Geometry: final body of the model. Coordinates: model frame, mm. Face numbers are marked on the shaded views. A direction names the side the tool comes from. Give positions to 0.01 mm unless a question says otherwise; leave off trailing zeros. Order: outer loops, then holes, each group sorted by start corner. A loop starts at its lowest first (then second) coordinate and runs counter-clockwise, first axis right, second up. Notation, with made-up numbers: (71, -13) - (83, -13) arc R7 ccw to (83, 0) - close; hole circle Ø7 at (27, 60). An arc over 180 degrees is marked (long way). Put each result on its own line as item: value. Start each with the question number.
1. Section B-B on z = 6. Return the cut outline in (x, y).
2. Section C-C on x = -807.5. Return the cut outline in (y, z).
3. Section A-A on y = -61. Return the cut outline in (x, z).
4. Ray query, line 1 along X through (y, z) = (-70.5, -0.5); line 2 along Y through (x, z) = (-773, -41); line 3 along Y through (x, z) = (-830, -5). Return the intervals inside material, ascending. Write a range as from..to.
5. Set-up query: the marked faces 5, 6, 7 and 8. Return all of +Z, -Z, +X, -X, +Y, -Y with unobstructed straight access to the full face (end or side cutting, diameter ignored); none if empty.
6. Section D-D on z = 31. Return the cut outline in (x, y), plus the area to 3 significant figures.
7. First-contact query: P1, Ø5, axis at y = -16.5, z = 34.5, coming from the +X side; P2, Ø4, axis at y = -11, z = 44.5, coming from the +X side; P3, Ø7, axis at x = -791.5, y = -61, coming from the -Z side; P4, Ø11.5, axis at y = -53.5, z = -4, coming from the +X side. Flat tips, straight axial feed; report the tip coordinate or a pass-through.
8. Mould query, pull axis X, two halves, no side actions, for the marked faces 1, 2, 3 and 4. Classes: pulls with the +X half, pulls with the -X half, needs draft (parallel to the pull), parting line crosses it, or undercut.
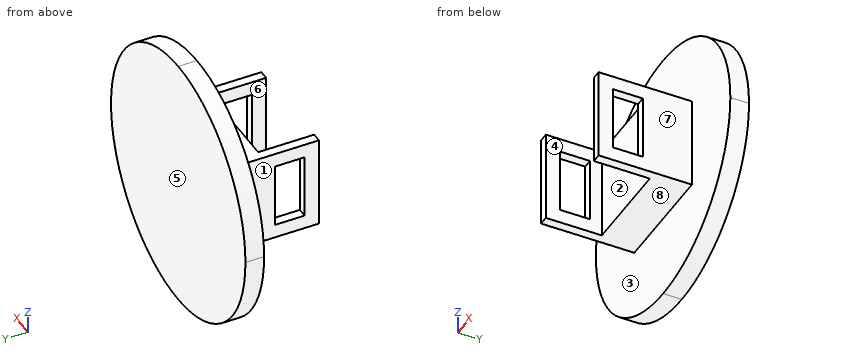
from build123d import *

# Parameters (mm, degrees)
F1_DEPTH = 12.7
F0_W     = 6.35
F0_H     = 31.75
F2_DEPTH = 76.2
F0_W_2   = 31.75
F3_DEPTH = 38.1
F4_W     = 20.32
F4_H     = 44.45
F5_DEPTH = 200.02717


with BuildPart() as f1:
    # F0 (on Front) → F1 (new body)
    with BuildSketch(Plane.XZ):
        with BuildLine():
            Line((-789.6218383789, 3.1863217354), (-738.8218383789, 3.1863217354))
            ThreePointArc((-738.8218383789, 3.1863217354), (-764.8600455314, 66.0481145829), (-827.7218383789, 92.0863217354))
            Line((-827.7218383789, 92.0863217354), (-827.7218383789, 34.9363217354))
            Line((-827.7218383789, 34.9363217354), (-795.9718383789, 34.9363217354))
            Line((-795.9718383789, 34.9363217354), (-789.6218383789, 34.9363217354))
            Line((-789.6218383789, 34.9363217354), (-789.6218383789, 3.1863217354))
        make_face()
        with BuildLine():
            Line((-827.7218383789, 34.9363217354), (-827.7218383789, 92.0863217354))
            ThreePointArc((-827.7218383789, 92.0863217354), (-890.5836312264, 66.0481145829), (-916.6218383789, 3.1863217354))
            Line((-916.6218383789, 3.1863217354), (-865.8218383789, 3.1863217354))
            Line((-865.8218383789, 3.1863217354), (-865.8218383789, 34.9363217354))
            Line((-865.8218383789, 34.9363217354), (-859.4718383789, 34.9363217354))
            Line((-859.4718383789, 34.9363217354), (-827.7218383789, 34.9363217354))
        make_face()
        with BuildLine():
            ThreePointArc((-916.6218383789, 3.1863217354), (-890.5836312264, -59.6754711121), (-827.7218383789, -85.7136782646))
            Line((-827.7218383789, -85.7136782646), (-827.7218383789, -28.5636782646))
            Line((-827.7218383789, -28.5636782646), (-859.4718383789, -28.5636782646))
            Line((-859.4718383789, -28.5636782646), (-865.8218383789, -28.5636782646))
            Line((-865.8218383789, -28.5636782646), (-865.8218383789, 3.1863217354))
            Line((-865.8218383789, 3.1863217354), (-916.6218383789, 3.1863217354))
        make_face()
        with BuildLine():
            ThreePointArc((-827.7218383789, -85.7136782646), (-764.8600455314, -59.6754711121), (-738.8218383789, 3.1863217354))
            Line((-738.8218383789, 3.1863217354), (-789.6218383789, 3.1863217354))
            Line((-789.6218383789, 3.1863217354), (-789.6218383789, -28.5636782646))
            Line((-789.6218383789, -28.5636782646), (-795.9718383789, -28.5636782646))
            Line((-795.9718383789, -28.5636782646), (-827.7218383789, -28.5636782646))
            Line((-827.7218383789, -28.5636782646), (-827.7218383789, -85.7136782646))
        make_face()
    extrude(amount=F1_DEPTH)

    # F0 (on Front) → F2 (join)
    with BuildSketch(Plane.XZ):
        with Locations((-862.6468383789, -12.6886782646)):
            Rectangle(F0_W, F0_H)
        with Locations((-862.6468383789, 19.0613217354)):
            Rectangle(F0_W, F0_H)
        with Locations((-792.7968383789, -12.6886782646)):
            Rectangle(F0_W, F0_H)
        with Locations((-792.7968383789, 19.0613217354)):
            Rectangle(F0_W, F0_H)
    extrude(amount=F2_DEPTH)

    # F0 (on Front) → F3 (join)
    with BuildSketch(Plane.XZ):
        with Locations((-811.8468383789, -12.6886782646)):
            Rectangle(F0_W_2, F0_H)
        with Locations((-843.5968383789, -12.6886782646)):
            Rectangle(F0_W_2, F0_H)
        with Locations((-843.5968383789, 19.0613217354)):
            Rectangle(F0_W_2, F0_H)
        with Locations((-811.8468383789, 19.0613217354)):
            Rectangle(F0_W_2, F0_H)
    extrude(amount=F3_DEPTH)

    # F4 (on face) → F5 (cut)
    with BuildSketch(Plane.YZ.offset(-789.6218383789)):
        with Locations((-56.2796956563, 3.1863217354)):
            Rectangle(F4_W, F4_H)
    extrude(amount=-F5_DEPTH, mode=Mode.SUBTRACT)


solid = f1.part
Resolved:
1. outline: (-916.58, -12.7) - (-865.82, -12.7) - (-865.82, -46.12) - (-859.47, -46.12) - (-859.47, -38.1) - (-795.97, -38.1) - (-795.97, -46.12) - (-789.62, -46.12) - (-789.62, -12.7) - (-738.87, -12.7) - (-738.87, 0) - (-916.58, 0) - close; (-865.82, -76.2) - (-859.47, -76.2) - (-859.47, -66.44) - (-865.82, -66.44) - close; (-795.97, -76.2) - (-789.62, -76.2) - (-789.62, -66.44) - (-795.97, -66.44) - close
2. outline: (-38.1, -28.56) - (-12.7, -28.56) - (-12.7, -83.38) - (0, -83.38) - (0, 89.76) - (-12.7, 89.76) - (-12.7, 34.94) - (-38.1, 34.94) - close
3. outline: (-865.82, -28.56) - (-859.47, -28.56) - (-859.47, -19.04) - (-865.82, -19.04) - close; (-865.82, 25.41) - (-859.47, 25.41) - (-859.47, 34.94) - (-865.82, 34.94) - close; (-795.97, -28.56) - (-789.62, -28.56) - (-789.62, -19.04) - (-795.97, -19.04) - close; (-795.97, 25.41) - (-789.62, 25.41) - (-789.62, 34.94) - (-795.97, 34.94) - close
4. line 1: -865.82..-859.47, -795.97..-789.62
4. line 2: -12.7..0
4. line 3: -38.1..0
5. face 5: +Z, -Z, +X, -X, +Y
5. face 6: +Z, -Z, -Y
5. face 7: +Z, -Z, +X, -Y
5. face 8: -Z, +X, -X, -Y
6. outline: (-912.16, -12.7) - (-865.82, -12.7) - (-865.82, -76.2) - (-859.47, -76.2) - (-859.47, -38.1) - (-795.97, -38.1) - (-795.97, -76.2) - (-789.62, -76.2) - (-789.62, -12.7) - (-743.28, -12.7) - (-743.28, 0) - (-912.16, 0) - close
6. area: 4,560 mm^2
7. P1: x = -789.62
7. P2: x = -747.99
7. P3: z = -28.56
7. P4: through
8. face 1: pulls with the -X half
8. face 2: undercut
8. face 3: needs draft
8. face 4: undercut
